Verification items for the finished model (mm, model axes). A direction names the side the tool comes from. Give positions to 0.01 mm unless a question says otherwise; leave off trailing zeros. Order: outer loops, then holes, each group sorted by start corner. A loop starts at its lowest first (then second) coordinate and runs counter-clockwise, first axis right, second up.
(1) Sectioned sample at D-D on z = 14. Count the separate pieces of the cut face and the enclosed holes in it, plus the area to 3 significant figures.
(2) Sectioned sample at B-B on y = -3.5. Record the cut outline in (x, z).
(3) Gauge pin test, flat ends, axial feed: pin 1 (15.5 mm diameter, centred on x = 2.5, y = -4, fed in from +Z); pin 2 (12 mm diameter, centred on x = -14.5, y = -9, fed in from -Z); pin 3 (6 mm diameter, centred on x = 0.5, y = -4.5, fed in from +Z); pin 4 (0.9 mm diameter, centred on x = 25.5, y = -9, fed in from +Z). Record the tip position at first contact, or that the pin passes through.
(4) Scan lines: L1, parallel to Y at x = 25.8, z = 13.55; L2, parallel to Y at x = 4.5, z = 9.25; L3, parallel to X at y = 9.5, z = 12. Record each from-to range of solid material in increasing order.
(5) Sectioned sample at A-A on x = -19.5. Record the cut outline in (y, z).
(6) Mould release check, pull along Z, two halves, no side actions. Record for faces 5 (the face through (25.68, -8.26, 14.36)), 6 (the face through (-27.79, 3.77, 9.85)), 7 (the face through (-3, 10, 3)): pulls with the +Z half, pulls with the -Z half, needs draft (parallel to the pull), parting line crosses it, or undercut.
(7) Access from +Z, -Z, +X, -X, +Y, -Y to the whole of each face (thin tool, end or side, straight path). Record for faces 1 (the face through (-27.79, -6.17, 13.35)), 2 (the face through (28.8, 0, 10)), 3 (the face through (-26.75, 0, 10)), 4 (the face through (15.813, -8.541, 2.423)).
(8) Sectioned sample at C-C on x = 3.5. Record the cut outline in (y, z).
Solid Edge part; units mm, degrees
sketch "Sketch1" plane through (0, 0, 0) normal (0, 0, 1) x (1, 0, 0)
  line L0 (-26.75, -15.6) -> (26.75, -15.6)
  line L1 (26.75, -15.6) -> (26.75, 15.6)
  line L2 (26.75, 15.6) -> (-26.75, 15.6)
  line L3 (-26.75, 15.6) -> (-26.75, -15.6)
extrude "Protrusion1" add sketch "Sketch1" along normal blind 3
sketch "Sketch2" plane through (0, 0, 0) normal (0, 0, 1) x (1, 0, 0)
  line L0 (-26.75, -15.6) -> (26.75, -15.6)
  line L1 (26.75, -15.6) -> (26.75, 15.6)
  line L2 (26.75, 15.6) -> (-26.75, 15.6)
  line L3 (-26.75, 15.6) -> (-26.75, -15.6)
  line L4 (-25.8, -17.1) -> (25.8, -17.1)
  arc A0 (28.8, -14.1) -> (25.8, -17.1) centre (25.8, -14.1) cw
  line L5 (28.8, -14.1) -> (28.8, 14.1)
  arc A1 (25.8, 17.1) -> (28.8, 14.1) centre (25.8, 14.1) cw
  line L6 (25.8, 17.1) -> (-25.8, 17.1)
  arc A2 (-28.8, 14.1) -> (-25.8, 17.1) centre (-25.8, 14.1) cw
  line L7 (-28.8, 14.1) -> (-28.8, -14.1)
  arc A3 (-28.8, -14.1) -> (-25.8, -17.1) centre (-25.8, -14.1) ccw
extrude "Wyciągnięcie_2" add sketch "Sketch2" along normal blind 15
chamfer "Faza_4" distance 1 angle 45 8 edges at (28.8, 0, 0) (27.9213, 16.2213, 0) (0, 17.1, 0) (-27.9213, 16.2213, 0) (-28.8, 0, 0) (-27.9213, -16.2213, 0) (0, -17.1, 0) (27.9213, -16.2213, 0)
sketch "Sketch3" plane through (0, 0, 3) normal (0, 0, 1) x (1, 0, 0)
  line L0 (26.75, 15.6) -> (22.07, 15.6)
  line L1 (22.07, 15.6) -> (22.07, -15.6)
  line L2 (22.07, -15.6) -> (26.75, -15.6)
  line L3 (26.75, -15.6) -> (26.75, 15.6)
extrude "Wycięcie_2" add sketch "Sketch3" along normal blind 12
sketch "Sketch4" plane through (-28.8, 0, 8) normal (-1, 0, 0) x (0, -1, 0)
  line L0 (-2.208, 2.2848) -> (4.6031, 2.2848)
  arc A0 (5.7031, 3.3848) -> (4.6031, 2.2848) centre (4.6031, 3.3848) cw
  line L1 (5.7031, 3.3848) -> (5.7031, 3.8218)
  arc A1 (4.6031, 4.9218) -> (5.7031, 3.8218) centre (4.6031, 3.8218) cw
  line L2 (4.6031, 4.9218) -> (-2.208, 4.9218)
  arc A2 (-2.208, 4.9218) -> (-3.308, 3.8218) centre (-2.208, 3.8218) ccw
  line L3 (-3.308, 3.8218) -> (-3.308, 3.3848)
  arc A3 (-3.308, 3.3848) -> (-2.208, 2.2848) centre (-2.208, 3.3848) ccw
extrude "Wycięcie_3" cut sketch "Sketch4" against normal blind 11.9554
sketch "Sketch5" plane through (-2.34, 0, 3) normal (0, 0, 1) x (1, 0, 0)
  line L0 (-24.41, 15.6) -> (-24.41, 15.2)
  line L1 (-24.41, 15.2) -> (24.41, 15.2)
  line L2 (24.41, 15.2) -> (24.41, 15.6)
  line L3 (24.41, 15.6) -> (-24.41, 15.6)
extrude "Wyciągnięcie_4" add sketch "Sketch5" along normal blind 12
sketch "Sketch6" plane through (-0.1019, 0, 15) normal (0, 0, 1) x (1, 0, 0)
  line L0 (-25.6981, -17.1) -> (25.9019, -17.1)
  arc A0 (25.9019, -17.1) -> (28.9019, -14.1) centre (25.9019, -14.1) ccw
  line L1 (28.9019, -14.1) -> (28.9019, 14.1)
  arc A1 (25.9019, 17.1) -> (28.9019, 14.1) centre (25.9019, 14.1) cw
  line L2 (25.9019, 17.1) -> (-25.6981, 17.1)
  arc A2 (-28.6981, 14.1) -> (-25.6981, 17.1) centre (-25.6981, 14.1) cw
  line L3 (-28.6981, 14.1) -> (-28.6981, -14.1)
  arc A3 (-28.6981, -14.1) -> (-25.6981, -17.1) centre (-25.6981, -14.1) ccw
  line L4 (-26.6481, 15.2) -> (22.1719, 15.2)
  line L5 (22.1719, 15.2) -> (22.1719, -15.6)
  line L6 (22.1719, -15.6) -> (-26.6481, -15.6)
  line L7 (-26.6481, -15.6) -> (-26.6481, 15.2)
extrude "Wyciągnięcie_5" add sketch "Sketch6" along normal blind 3
sketch "Sketch7" plane through (0, 0, 18) normal (0, 0, 1) x (1, 0, 0)
  line L0 (-26.75, -15.6) -> (-26.75, -16.1)
  line L1 (-26.75, -16.1) -> (22.0731, -16.1)
  line L2 (22.0731, -16.1) -> (22.07, -15.6)
  line L3 (22.07, -15.6) -> (-26.75, -15.6)
extrude "Wycięcie_6" cut sketch "Sketch7" against normal blind 15
sketch "Sketch8" plane through (0, 0, 18) normal (0, 0, 1) x (1, 0, 0)
  circle A0 centre (25.8, 9.15) radius 0.9
  circle A1 centre (25.8, -9.15) radius 0.9
extrude "Wycięcie_7" cut sketch "Sketch8" against normal blind 6.6184
sketch "Sketch9" plane through (-2.3384, -0.45, 3) normal (0, 0, 1) x (-1, 0, 0)
  line L0 (-24.4116, 15.65) -> (-24.1616, 15.65)
  line L1 (-24.1616, 15.65) -> (-24.1616, -15.65)
  line L2 (-24.1616, -15.65) -> (-24.4084, -15.65)
  line L3 (-24.4084, -15.65) -> (-24.4116, 15.65)
extrude "Wyciągnięcie_6" add sketch "Sketch9" along normal blind 15
sketch "Sketch10" plane through (0, 0, 18) normal (0, 0, 1) x (-1, 0, 0)
  line L0 (-38.4633, -19.2005) -> (38.4633, -19.2005)
  line L1 (38.4633, -19.2005) -> (38.4633, 19.2005)
  line L2 (38.4633, 19.2005) -> (-38.4633, 19.2005)
  line L3 (-38.4633, 19.2005) -> (-38.4633, -19.2005)
extrude "Wycięcie_9" cut sketch "Sketch10" against normal blind 0.75
sketch "Sketch11" plane through (0, 0, 0) normal (0, 0, -1) x (1, 0, 0)
  line L0 (-34.3065, -19.3102) -> (34.3065, -19.3102)
  line L1 (34.3065, -19.3102) -> (34.3065, 19.3102)
  line L2 (34.3065, 19.3102) -> (-34.3065, 19.3102)
  line L3 (-34.3065, 19.3102) -> (-34.3065, -19.3102)
extrude "Wycięcie_10" cut sketch "Sketch11" against normal blind 2
chamfer "Faza_13" distance 1 angle 45 8 edges at (-28.8, 0, 2) (-27.9213, 16.2213, 2) (0, 17.1, 2) (27.9213, 16.2213, 2) (28.8, 0, 2) (27.9213, -16.2213, 2) (0, -17.1, 2) (-27.9213, -16.2213, 2)
sketch "Sketch12" plane through (0, 0, 17.25) normal (0, 0, 1) x (-1, 0, 0)
  line L0 (-21.8231, -15.2) -> (-21.8231, -14.7)
  line L1 (-21.8231, -14.7) -> (26.75, -14.7)
  line L2 (26.75, -14.7) -> (26.75, -15.2)
  line L3 (26.75, -15.2) -> (-21.8231, -15.2)
extrude "Protrusion2" add sketch "Sketch12" against normal up to vertex (14.25 mm away)
sketch "Sketch13" plane through (0, 0, 2) normal (0, 0, -1) x (1, 0, 0)
  line L0 (-14.9, 8.6489) -> (14.9, 8.6478)
  arc A0 (14.9, 8.6478) -> (15.9, 7.6478) centre (14.9, 7.6478) cw
  line L1 (15.9, 7.6478) -> (15.9, -6.9988)
  arc A1 (14.9, -7.9988) -> (15.9, -6.9988) centre (14.9, -6.9988) ccw
  line L2 (14.9, -7.9988) -> (-14.9006, -7.9988)
  arc A2 (-15.9006, -6.9988) -> (-14.9006, -7.9988) centre (-14.9006, -6.9988) ccw
  line L3 (-15.9, 7.649) -> (-15.9006, -6.9988)
  arc A3 (-15.9, 7.649) -> (-14.9, 8.6489) centre (-14.9, 7.6489) cw
extrude "Wyciągnięcie_8" cut sketch "Sketch13" against normal blind 166.3187
chamfer "Faza_16" distance 2.1 angle 45 8 edges at (-28.8, -1.1976, 10.2848) (-28.8, -5.381, 10.6069) (-28.8, -5.7031, 11.6033) (-28.8, -5.381, 12.5996) (-28.8, -1.1976, 12.9218) (-28.8, 2.9858, 12.5996) (-28.8, 3.308, 11.6033) (-28.8, 2.9858, 10.6069)
chamfer "Faza_17" distance 0.7 angle 45 8 edges at (-0.0003, 7.9988, 2) (-15.6077, 7.7059, 2) (-15.9003, -0.3251, 2) (-15.6071, -8.3561, 2) (0, -8.6484, 2) (15.6071, -8.3549, 2) (15.9, -0.3245, 2) (15.6071, 7.7059, 2)
Ans:
1. separate pieces: 1
1. enclosed holes: 3
1. area: 451 mm2
2. outline: (-28.8, 3) - (-27.8, 2) - (-16.6, 2) - (-15.9, 2.7) - (-15.9, 3) - (-26.75, 3) - (-26.75, 10.23) - (-28.8, 8.18) - close; (-28.8, 15.02) - (-26.75, 12.97) - (-26.75, 17.25) - (-28.8, 17.25) - close; (15.9, 2.7) - (16.6, 2) - (27.8, 2) - (28.8, 3) - (28.8, 17.25) - (21.82, 17.25) - (21.82, 3) - (15.9, 3) - close
3. pin 1: stops at z = 3
3. pin 2: stops at z = 2
3. pin 3: passes through
3. pin 4: stops at z = 11.38
4. L1: y = -17.1 to -10.05, -8.25 to 8.25, 10.05 to 17.1
4. L2: y = -17.1 to -16.1, 14.7 to 17.1
4. L3: x = -28.8 to -26.75, 21.82 to 24.97, 26.63 to 28.8
5. outline: (-17.1, 3) - (-16.1, 2) - (16.1, 2) - (17.1, 3) - (17.1, 17.25) - (14.7, 17.25) - (14.7, 3) - (-16.1, 3) - (-16.1, 17.25) - (-17.1, 17.25) - close
6. face 5: needs draft
6. face 6: undercut
6. face 7: pulls with the +Z half
7. face 1: -X
7. face 2: +Z, -Z, +X, +Y, -Y
7. face 3: +Z
7. face 4: -Z
8. outline: (-17.1, 3) - (-16.1, 2) - (-9.35, 2) - (-8.65, 2.7) - (-8.65, 3) - (-16.1, 3) - (-16.1, 17.25) - (-17.1, 17.25) - close; (8, 2.7) - (8.7, 2) - (16.1, 2) - (17.1, 3) - (17.1, 17.25) - (14.7, 17.25) - (14.7, 3) - (8, 3) - close
